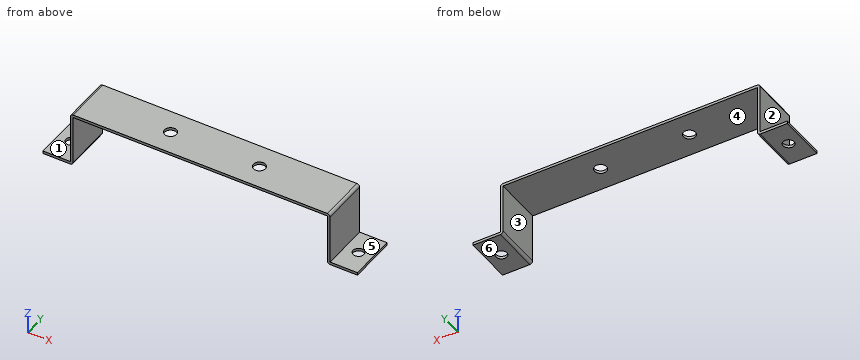
```python
from build123d import *

# Parameters (mm, degrees)
F1_DEPTH = 17.5
F2_R     = 4
F3_DEPTH = 25
F4_R     = 4.4
F5_DEPTH = 25
F6_R     = 2


# Not quite as in the source:
# - a feature names something its author has since deleted; it is built from what else it names


with BuildPart() as f1:
    # F0 (on Front) → F1 (new body, symmetric)
    with BuildSketch(Plane.XZ):
        Polygon((95, -38), (95, 0), (-95, 0), (-95, -38), (-115, -38), (-115, -40), (-93, -40), (-93, -2), (93, -2), (93, -40), (115, -40), (115, -38), align=None)
    extrude(amount=F1_DEPTH, both=True)

    # F2 (on face) → F3 (cut)
    with BuildSketch(Plane.XY.offset(-38)):
        with Locations((-105, 0)):
            Circle(F2_R)
        with Locations((105, 0)):
            Circle(F2_R)
    extrude(amount=-F3_DEPTH, mode=Mode.SUBTRACT)

    # F4 (on face) → F5 (cut)
    with BuildSketch(Plane.XY):
        with Locations((-32.5, 0)):
            Circle(F4_R)
        with Locations((32.5, 0)):
            Circle(F4_R)
    extrude(amount=-F5_DEPTH, mode=Mode.SUBTRACT)

    # F6
    f6_edges = [f1.edges().sort_by_distance(p)[0] for p in [
        (95, 0, 0),
        (-95, 0, 0),
        (-93, 0, -40),
        (93, 0, -40),
    ]]
    fillet(f6_edges, radius=F6_R)


solid = f1.part
```
Work out the finished part from the listing and answer in its coordinate system (mm). Face numbers are marked on the shaded views. A direction names the side the tool comes from. Round coordinates to 2 decimals unless told otherwise and drop trailing zeros. Loops run counter-clockwise (first coordinate to the right, second up) from the corner with the lowest first, then second, coordinate; pieces in that order, holes last. Notation, with made-up numbers: (-16.5, 31.25) -> (4.5, 31.25) arc R15 cw to (4.5, 52.25) -> close; hole circle Ø4 at (82, 20). An arc over 180 degrees is marked (long way). Write each question's results on one line, items separated by ' | '. Start each with the question number.
1. For a pull along X with two mould halves and no side action, classify the marked faces 1, 2 and 3 as +X half, -X half, draft (parallel to the pull), parting line (faces both ways), or undercut.
2. A tool of negligible diameter and unlimited length cuts with its end or side. For the marked faces 4, 5 and 6, from which of +Z, -Z, +X, -X, +Y, -Y can it reach the whole face along a straight path? Write none if from no direction.
3. Section C-C (y = -7) is taken. Determine the outline of the cut face in (x, z), plus the area to 3 significant figures.
4. Given pin 1 Ø1 at (y, z) = (-13.5, -31.5) entering from -X; pin 2 Ø17.5 at (y, z) = (5, -13) entering from +X; pin 3 Ø6 at (x, y) = (-108.5, 7) entering from +Z, each flat-ended and moving along its own axis, determine where each tip first touches the part or whether it passes through.
5. Find the intervals of material crossed by probe 1 along X at (y, z) = (2, -16); probe 2 along Y at (x, z) = (105, -39.4); probe 3 along Y at (x, z) = (32.5, -0.45), in increasing order. Write a range as from..to.
6. Section A-A (z = -32.5) is taken. Determine the outline of the cut face in (x, y), plus the area to 3 significant figures.
7. Section D-D (x = -9.5) is taken. Determine the outline of the cut face in (y, z), plus the area to 3 significant figures.
8. Section B-B (x = -105) is taken. Determine the outline of the cut face in (y, z).
Evaluation:
1) face 1: draft | face 2: -X half | face 3: undercut
2) face 4: -Z, +Y, -Y | face 5: +Z, +X, +Y, -Y | face 6: -Z, +X, -X, +Y, -Y
3) outline: (-115, -40) -> (-95, -40) arc R2 ccw to (-93, -38) -> (-93, -2) -> (93, -2) -> (93, -38) arc R2 ccw to (95, -40) -> (115, -40) -> (115, -38) -> (95, -38) -> (95, -2) arc R2 ccw to (93, 0) -> (-93, 0) arc R2 ccw to (-95, -2) -> (-95, -38) -> (-115, -38) -> close | area: 609 mm2
4) pin 1: stops at x = -95 | pin 2: stops at x = 95 | pin 3: stops at z = -38
5) probe 1: x = -95..-93, 93..95 | probe 2: y = -17.5..-4, 4..17.5 | probe 3: y = -17.5..-4.4, 4.4..17.5
6) outline: (-95, -17.5) -> (-93, -17.5) -> (-93, 17.5) -> (-95, 17.5) -> close; (93, -17.5) -> (95, -17.5) -> (95, 17.5) -> (93, 17.5) -> close | area: 140 mm2
7) outline: (-17.5, -2) -> (17.5, -2) -> (17.5, 0) -> (-17.5, 0) -> close | area: 70.0 mm2
8) outline: (-17.5, -40) -> (-4, -40) -> (-4, -38) -> (-17.5, -38) -> close; (4, -40) -> (17.5, -40) -> (17.5, -38) -> (4, -38) -> close
